Check sheet for the drawn part. Datum: minimum x, y, z corner. Units: mm. A direction names the side the tool comes from. Coordinates: 2 decimals unless noted, no trailing zeros. Write each loop counter-clockwise with the first axis right and the second up, starting at its lowest first coordinate (ties: lowest second). Pieces come first, ordered by that corner, then holes. Notation, with made-up numbers: (1, -11.5) - (37, -11.5) arc R33 ccw to (37, 21.5) - close; hole circle Ø10 at (-23.5, -25.75). An arc over 180 degrees is marked (long way). Write each question's results on one line, items separated by ' | '.
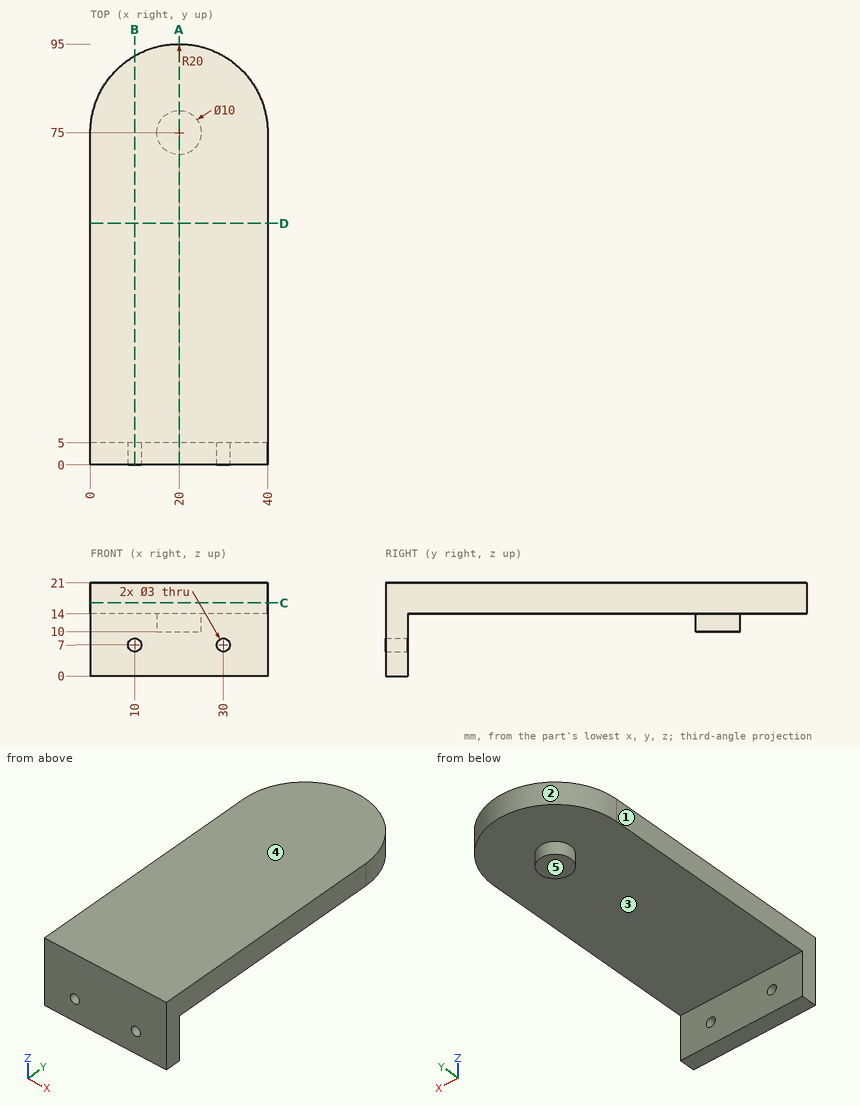
1. Sectioned sample at A-A (x = 20). Record the cut outline in (y, z), then the cut area to 3 significant figures.
Values follow:
outline: (0, 0) - (5, 0) - (5, 14) - (70, 14) - (70, 10) - (80, 10) - (80, 14) - (95, 14) - (95, 21) - (0, 21) - close | area: 775 mm^2
2. Draft check along Y on the marked faces 1, 2 and 3. Enter one of: pulls with the +Y half, pulls with the -Y half, needs draft (parallel to the pull), parting line crosses it, or undercut.
Values follow:
face 1: needs draft | face 2: pulls with the +Y half | face 3: undercut
3. Sectioned sample at D-D (y = 54.5). Record the cut outline in (x, z), then the cut area to 3 significant figures.
Values follow:
outline: (0, 14) - (40, 14) - (40, 21) - (0, 21) - close | area: 280 mm^2
4. Go/stop test with flat-tipped pins: pin 1 (2 mm diameter, centred on x = 9.5, z = 7.5, fed in from +Y); pin 2 (4 mm diameter, centred on x = 35.5, z = 18, fed in from +Y); pin 3 (2 mm diameter, centred on x = 17.5, y = 42, fed in from -Z). Record where each tip stops, or that it passes through.
Values follow:
pin 1: stops at y = 5 | pin 2: stops at y = 89.76 | pin 3: stops at z = 14
5. Material ranges on L1, parallel to X at y = 2.35, z = 7; L2, parallel to Z at x = 30, y = 1.1; L3, parallel to Z at x = 14, y = 77, recorded low to high. Write a range as [from, to].
Values follow:
L1: x = [0, 8.5], [11.5, 28.5], [31.5, 40] | L2: z = [0, 5.5], [8.5, 21] | L3: z = [14, 21]
6. Sectioned sample at B-B (x = 10). Record the cut outline in (y, z).
Values follow:
outline: (0, 0) - (5, 0) - (5, 5.5) - (0, 5.5) - close; (0, 8.5) - (5, 8.5) - (5, 14) - (92.32, 14) - (92.32, 21) - (0, 21) - close
7. Access from +Z, -Z, +X, -X, +Y, -Y to the whole of each face (thin tool, end or side, straight path). Record for the marked faces 4 and 5.
Values follow:
face 4: +Z, +X, -X, +Y, -Y | face 5: -Z, +X, -X, +Y
8. Sectioned sample at C-C (z = 16.5). Record the cut outline in (x, y).
Values follow:
outline: (0, 0) - (40, 0) - (40, 75) arc R20 ccw to (0, 75) - close
